Can you work these out from the model? Positions are in its coordinate system, mm. Coordinates: 2 decimals unless noted, no trailing zeros. Order: outer loops, then holes, each group sorted by start corner. A loop starts at its lowest first (then second) coordinate and runs counter-clockwise, first axis right, second up. Notation, with made-up numbers: (12.5, 42.25) -> (20.5, 42.25) arc R15 cw to (20.5, 66.25) -> close; hole circle Ø7 at (82, -3). An arc over 180 degrees is marked (long way). Use a Markdown table: item, result. Add a question column.
1. Suppose I cut it at B-B, the plane z = 3.5. List the corners of the cut face in (x, y) for me, then the cut area to 3 significant figures.
2. For pin 1 Ø8 at (y, z) = (4.5, 27) entering from -X; pin 2 Ø5 at (y, z) = (6.5, 15) entering from -X; pin 3 Ø6 at (y, z) = (-3.5, 20) entering from +X, each with a flat end and sliding along its axis, tell me the tip position at first contact or that it passes through.
3. Suppose I cut it at C-C, the plane z = 14. List the corners of the cut face in (x, y) for me, then the cut area to 3 significant figures.
4. Suppose I cut it at A-A, the plane x = 0. List the corners of the cut face in (y, z) for me, then the cut area to 3 significant figures.
5. If I drill on line 1 along X through (y, z) = (-5, 11); line 2 along Y through (x, z) = (-9, 4); line 3 along Y through (x, z) = (2.5, 16), over which ranges is the centre line in solid material (lowest first)? Write a range as from..to.
```python
from build123d import *

# Parameters (mm, degrees)
F0_R      = 11.013281
F1_DEPTH  = 6.35
F2_R      = 1.27
F1_FACE_R = 9.743281
F4_R      = 7.366


with BuildPart() as f1:
    # F0 (on Top) → F1 (new body)
    with BuildSketch(Plane.XY):
        Circle(F0_R)
    extrude(amount=F1_DEPTH)

    # F2
    f2_edges = [f1.edges().sort_by_distance(p)[0] for p in [
        (-11.013281, 0, 6.35),
        (-11.013281, 0, 0),
    ]]
    fillet(f2_edges, radius=F2_R)

    # F1_face (on face) → F5 section 0
    with BuildSketch(Plane.XY.offset(6.35)):
        Circle(F1_FACE_R)
    # F4 (on offset) → F5 section 1
    with BuildSketch(Plane.XY.offset(31.75)):
        Circle(F4_R)
    loft()


solid = f1.part
```
Worked out:
| question | item | result |
|---|---|---|
| 1 | outline | circle Ø22.03 at (0, 0) |
| 1 | area | 381 mm² |
| 2 | pin 1 | stops at x = -7.93 |
| 2 | pin 2 | stops at x = -8.02 |
| 2 | pin 3 | stops at x = 8.56 |
| 3 | outline | circle Ø18.05 at (0, 0) |
| 3 | area | 256 mm² |
| 4 | outline | (-11.01, 1.27) arc R1.27 ccw to (-9.74, 0) -> (9.74, 0) arc R1.27 ccw to (11.01, 1.27) -> (11.01, 5.08) arc R1.27 ccw to (9.74, 6.35) -> (7.37, 31.75) -> (-7.37, 31.75) -> (-9.74, 6.35) arc R1.27 ccw to (-11.01, 5.08) -> close |
| 4 | area | 573 mm² |
| 5 | line 1 | x = -7.85..7.85 |
| 5 | line 2 | y = -6.35..6.35 |
| 5 | line 3 | y = -8.48..8.48 |
